The listing builds one solid part. Answer for the finished solid, in the listing's coordinates (mm). A direction names the side the tool comes from. Give positions to 0.01 mm unless a question says otherwise; leave off trailing zeros. Write each loop counter-clockwise with the first axis right and the second up, starting at its lowest first coordinate (ties: lowest second). Pieces come first, ordered by that corner, then holes. Notation, with made-up numbers: (-31, 73) -> (5, 73) arc R13 ccw to (5, 77) -> close; hole circle Ø11 at (62, 25). An arc over 180 degrees is marked (long way). One line per question, with ' | ' between items.
from build123d import *

# Parameters (mm, degrees)
IZIM1_W                     = 72
IZIM1_H                     = 72
Y_KSEKLIK_EKSTR_ZYON1_DEPTH = 100
KES_EKSTR_ZYON2_DEPTH       = 67
KES_EKSTR_ZYON2_DEPTH_BACK  = 90


with BuildPart() as part:
    # Çizim1 → Yükseklik-Ekstrüzyon1 (new body)
    with BuildSketch(Plane.XY):
        with BuildLine():
            Line((-36, 40), (36, 40))
            ThreePointArc((36, 40), (38.828427125, 38.828427125), (40, 36))
            Line((40, 36), (40, -36))
            ThreePointArc((40, -36), (38.828427125, -38.828427125), (36, -40))
            Line((36, -40), (-36, -40))
            ThreePointArc((-36, -40), (-38.828427125, -38.828427125), (-40, -36))
            Line((-40, -36), (-40, 36))
            ThreePointArc((-40, 36), (-38.828427125, 38.828427125), (-36, 40))
        make_face()
        Rectangle(IZIM1_W, IZIM1_H, mode=Mode.SUBTRACT)
    extrude(amount=Y_KSEKLIK_EKSTR_ZYON1_DEPTH)

    # Çizim4 → Kes-Ekstrüzyon2 (cut, two sides: drawn at the far end of the back side and taken through both)
    with BuildSketch(Plane(origin=(0, 0, 0), x_dir=(1, 0, 0), z_dir=(0, 1, 0)).offset(-KES_EKSTR_ZYON2_DEPTH_BACK)):
        Polygon((-40, 0), (40, -80), (40, 0), align=None)
    extrude(amount=KES_EKSTR_ZYON2_DEPTH + KES_EKSTR_ZYON2_DEPTH_BACK, mode=Mode.SUBTRACT)


solid = part.part
Item 1: Consider line 1 (Y direction, x = -35, z = 28); line 2 (X direction, y = 34, z = 10.5). Determine where each line is inside the solid, lowest interval first. Write a range as [from, to].
Answers below:
line 1: [-40, -36], [36, 40] | line 2: [-40, -36]
Item 2: Determine the mould class of faces 1 (the face through (-9, -36, 62)), 2 (the face through (-7, -40, 62)), 3 (the face through (-38.797, -38.859, 49.3)) for opening direction X: pulls with the +X half, pulls with the -X half, needs draft (parallel to the pull), parting line crosses it, or undercut.
Answers below:
face 1: undercut | face 2: needs draft | face 3: pulls with the -X half
Item 3: Flat-ended cylindrical pins translate along their axes: pin 1 (21.5 mm diameter, centred on y = -2.5, z = 64, fed in from +X); pin 2 (12 mm diameter, centred on x = 2, z = 26.5, fed in from -Y). Find the tip coordinate at first contact, or state that the pin passes through.
Answers below:
pin 1: x = -36 | pin 2: through
Item 4: Find section A-A (y = 3). Write down the section's boundary in (x, z).
Answers below:
outline: (-40, 0) -> (-36, 4) -> (-36, 100) -> (-40, 100) -> close; (36, 76) -> (40, 80) -> (40, 100) -> (36, 100) -> close
Item 5: Find section D-D (z = 94). Write down the section's boundary in (x, y), then the cut area to 3 significant figures.
Answers below:
outline: (-40, -36) arc R4 ccw to (-36, -40) -> (36, -40) arc R4 ccw to (40, -36) -> (40, 36) arc R4 ccw to (36, 40) -> (-36, 40) arc R4 ccw to (-40, 36) -> close; hole (-36, -36) -> (36, -36) -> (36, 36) -> (-36, 36) -> close | area: 1,200 mm²
Item 6: Find section C-C (z = 68). Write down the section's boundary in (x, y), then the cut area to 3 significant figures.
Answers below:
outline: (-40, -36) arc R4 ccw to (-36, -40) -> (28, -40) -> (28, -36) -> (-36, -36) -> (-36, 36) -> (28, 36) -> (28, 40) -> (-36, 40) arc R4 ccw to (-40, 36) -> close | area: 825 mm²
Item 7: A tool of negligible diameter and unlimited length cuts with its end or side. For faces 4 (the face through (-9, 36, 62)), 5 (the face through (3, -38, 100)), from which of +Z, -Z, +X, -X, +Y, -Y can it reach the whole face along a straight path? Write none if from no direction.
Answers below:
face 4: +Z, -Z | face 5: +Z, +X, -X, +Y, -Y
Item 8: Find section B-B (x = 17). Write down the section's boundary in (y, z).
Answers below:
outline: (-40, 57) -> (-36, 57) -> (-36, 100) -> (-40, 100) -> close; (36, 57) -> (40, 57) -> (40, 100) -> (36, 100) -> close
